Design review of the part built by this model. Coordinates are the model's own, in mm. Give positions to 0.01 mm unless a question says otherwise; leave off trailing zeros. Order: outer loops, then holes, each group sorted by start corner. A loop starts at its lowest first (then second) coordinate and runs counter-clockwise, first axis right, second up. Notation, with made-up numbers: (-4, -10) - (29, -10) arc R16 cw to (29, -5) - close; hole circle Ø3 at (-30, -17.75). An arc over 180 degrees is marked (long way). Write each question's results on one line, items separated by ' | '. Start each with the question number.
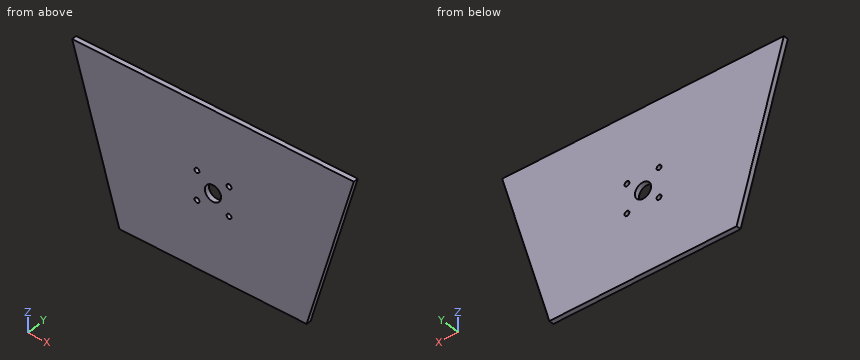
```python
from build123d import *

# Parameters (mm, degrees)
BOSS_EXTRUDE1_DEPTH        = 3
F_3_0MM_DOWEL_HOLE1_D      = 3
F_3_0MM_DOWEL_HOLE1_DEPTH  = 3
F_10_0MM_DOWEL_HOLE1_D     = 10
F_10_0MM_DOWEL_HOLE1_DEPTH = 3


with BuildPart() as part:
    # Sketch1 → Boss-Extrude1 (new body)
    with BuildSketch(Plane(origin=(0, 0, 0), x_dir=(1, 0, 0), z_dir=(0, 1, 0))):
        Polygon((5.2, 0), (180, 0), (150.720058283, 100), (34.479941717, 100), align=None)
    extrude(amount=BOSS_EXTRUDE1_DEPTH)

    # Ø3.0mm Dowel Hole1
    with Locations(Plane(origin=(0, 0, 0), x_dir=(-1, 0, 0), z_dir=(0, -1, 0))):
        with Locations((-82.65, 58.95), (-82.65, 41.05), (-102.55, 41.05), (-102.55, 58.95)):
            Hole(F_3_0MM_DOWEL_HOLE1_D / 2, depth=F_3_0MM_DOWEL_HOLE1_DEPTH)

    # Ø10.0mm Dowel Hole1
    with Locations(Plane(origin=(0, 3, 0), x_dir=(1, 0, 0), z_dir=(0, 1, 0))):
        with Locations((92.6, 50)):
            Hole(F_10_0MM_DOWEL_HOLE1_D / 2, depth=F_10_0MM_DOWEL_HOLE1_DEPTH)


solid = part.part
```
Q1. Add section D-D (z = -14.5). Give the boundary of the cut face in (x, y), plus the area to 3 significant figures.
Q2. Add section A-A (x = 92.6). Give the boundary of the cut face in (y, z).
Q3. Add section C-C (z = -50). Give the boundary of the cut face in (x, y).
Q4. Add section B-B (y = 2.15). Give the boundary of the cut face in (x, z).
Q5. For line 1 (Z direction, x = 102.55, y = 0.9); line 2 (X direction, y = 2.1, z = -41.05); line 3 (X direction, y = 0.6, z = -58.95), list the stretches that pass through material, from the lowest coordinate up. Write a range as [from, to].
Verdict:
1) outline: (9.45, 0) - (175.75, 0) - (175.75, 3) - (9.45, 3) - close | area: 499 mm2
2) outline: (0, -100) - (3, -100) - (3, -55) - (0, -55) - close; (0, -45) - (3, -45) - (3, 0) - (0, 0) - close
3) outline: (19.84, 0) - (87.6, 0) - (87.6, 3) - (19.84, 3) - close; (97.6, 0) - (165.36, 0) - (165.36, 3) - (97.6, 3) - close
4) outline: (5.2, 0) - (34.48, -100) - (150.72, -100) - (180, 0) - close; hole circle Ø3 at (82.65, -58.95); hole circle Ø3 at (82.65, -41.05); hole circle Ø10 at (92.6, -50); hole circle Ø3 at (102.55, -58.95); hole circle Ø3 at (102.55, -41.05)
5) line 1: z = [-100, -60.45], [-57.45, -42.55], [-39.55, 0] | line 2: x = [17.22, 81.15], [84.15, 101.05], [104.05, 167.98] | line 3: x = [22.46, 81.15], [84.15, 101.05], [104.05, 162.74]
